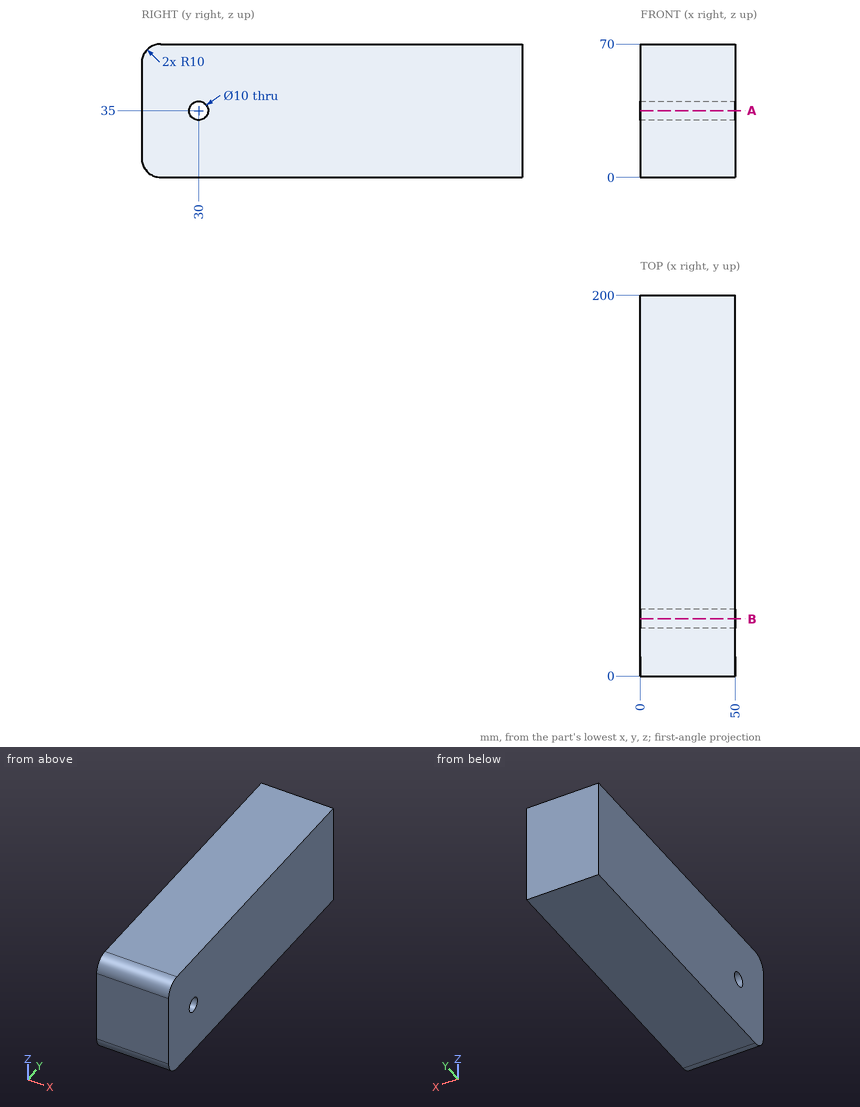
Here's the drawing with two shaded views (mm, measured from the low corner). I have some questions. Coordinates: 2 decimals unless noted, no trailing zeros. Order: outer loops, then holes, each group sorted by start corner. A loop starts at its lowest first (then second) coordinate and runs counter-clockwise, first axis right, second up.
Q1. Suppose I cut it at B-B on y = 30. Please give me the cut outline in (x, z), and give its area (3 significant figures).
Q2. Please list where this line runs through material, in increasing order: L1, parallel to Y at x = 15.5, z = 35.
Q3. Suppose I cut it at A-A on z = 35. Please give me the cut outline in (x, y), and give its area (3 significant figures).
Answer:
1. outline: (0, 0) - (50, 0) - (50, 30) - (0, 30) - close; (0, 40) - (50, 40) - (50, 70) - (0, 70) - close
1. area: 3,000 mm2
2. L1: y = 0 to 25, 35 to 200
3. outline: (0, 0) - (50, 0) - (50, 25) - (0, 25) - close; (0, 35) - (50, 35) - (50, 200) - (0, 200) - close
3. area: 9,500 mm2
